from build123d import *

# Parameters (mm, degrees)
SKETCH1_R                                        = 31
BOSS_EXTRUDE1_DEPTH                              = 17.78
CBORE_FOR_3_8_SOCKET_HEAD_CAP_SCREW1_D           = 9.8044
CBORE_FOR_3_8_SOCKET_HEAD_CAP_SCREW1_DEPTH       = 23.8252
CBORE_FOR_3_8_SOCKET_HEAD_CAP_SCREW1_CBORE_D     = 15.875
CBORE_FOR_3_8_SOCKET_HEAD_CAP_SCREW1_CBORE_DEPTH = 9.525
CBORE_FOR_3_8_SOCKET_HEAD_CAP_SCREW1_TIP         = 2.945538927
CHAMFER1_SIZE                                    = 0.762


with BuildPart() as part:
    # Sketch1 → Boss-Extrude1 (new body)
    with BuildSketch(Plane(origin=(0, 0, 0), x_dir=(0, 0, -1), z_dir=(1, 0, 0))):
        Circle(SKETCH1_R)
    extrude(amount=BOSS_EXTRUDE1_DEPTH)

    # CBORE for 3/8 Socket Head Cap Screw1
    with Locations(Plane(origin=(17.78, 0, 0), x_dir=(0, 0, -1), z_dir=(1, 0, 0))):
        with Locations((-15.24, 0), (15.24, 0)):
            CounterBoreHole(CBORE_FOR_3_8_SOCKET_HEAD_CAP_SCREW1_D / 2, CBORE_FOR_3_8_SOCKET_HEAD_CAP_SCREW1_CBORE_D / 2, CBORE_FOR_3_8_SOCKET_HEAD_CAP_SCREW1_CBORE_DEPTH, depth=CBORE_FOR_3_8_SOCKET_HEAD_CAP_SCREW1_DEPTH)
            with Locations((0, 0, -(CBORE_FOR_3_8_SOCKET_HEAD_CAP_SCREW1_DEPTH + CBORE_FOR_3_8_SOCKET_HEAD_CAP_SCREW1_TIP / 2))):  # 118° drill point
                Cone(0, CBORE_FOR_3_8_SOCKET_HEAD_CAP_SCREW1_D / 2, CBORE_FOR_3_8_SOCKET_HEAD_CAP_SCREW1_TIP, mode=Mode.SUBTRACT)

    # Chamfer1
    chamfer1_edges = [part.edges().sort_by_distance(p)[0] for p in [
        (17.78, 0, 23.1775),
        (0, 0, 31),
        (17.78, 0, 31),
        (17.78, 0, -7.3025),
    ]]
    chamfer(chamfer1_edges, length=CHAMFER1_SIZE)


solid = part.part
The model under review builds one solid part; all positions refer to its coordinate system, in mm. A direction names the side the tool comes from. Round coordinates to 2 decimals unless told otherwise and drop trailing zeros. Write each loop counter-clockwise with the first axis right and the second up, starting at its lowest first coordinate (ties: lowest second). Pieces come first, ordered by that corner, then holes. Notation, with made-up numbers: M -16,-4 L 11,-4 A24 cw 11,21 Z; hole C -25,25.25 d7. An arc over 180 degrees is marked long. Answer as CSV lines item,"result". Start each with the question number.
Q1. The part is to be moulded in two halves that separate along Z. For faces 1 (the face through (4.07, 0.216, -20.137)), 2 (the face through (17.78, 0, 0)), 3 (the face through (8.255, 4, 12)), 4 (the face through (8.776, 30.736, 4.036)), say which applies: +Z half, -Z half, draft (parallel to the pull), parting line (faces both ways), or undercut.
Q2. Tool access review of faces 5 (the face through (0, 0, 0)), 6 (the face through (12.698, -3.04, 7.908)): name each direction out of +Z, -Z, +X, -X, +Y, -Y from which nothing blocks a thin tool from reaching the whole face with its end or side.
Q3. Consider section A-A, the plane y = 0. Give the boundary of the cut face in (x, z) (1 decimal).
Q4. Consider section B-B, the plane x = 13.75. Give the boundary of the cut face in (y, z) (1 decimal).
Q5. Wall thickness on line 1 along Y through (x, z) = (14, 0); line 2 along Y through (x, z) = (5.5, -18); line 3 along Z through (x, y) = (7.75, -1): over which ranges is each line inside the solid? List them lowest first.
Q6. Clearance check with flat-ended pins moving along their axes: P1, Ø5, axis at x = 6.5, z = -3.5, coming from the +Y side; P2, Ø2, axis at x = 12, z = 21.5, coming from the +Y side; P3, Ø10, axis at x = 12.5, z = 15, coming from the +Y side. State where each tip first meets the part, or that it passes through.
Q7. Consider section C-C, the plane x = 4. Give the boundary of the cut face in (y, z), then the cut area to 3 significant figures.
Result set:
1,face 1,"undercut"
1,face 2,"draft"
1,face 3,"undercut"
1,face 4,"parting line"
2,face 5,"+Z, -Z, -X, +Y, -Y"
2,face 6,"+X"
3,outline,"M 0,-30.2 L 0.8,-31 L 17,-31 L 17.8,-30.2 L 17.8,-23.9 L 17,-23.2 L 8.3,-23.2 L 8.3,-20.1 L 0,-20.1 Z; M 0,-10.3 L 8.3,-10.3 L 8.3,-7.3 L 17,-7.3 L 17.8,-6.5 L 17.8,6.5 L 17,7.3 L 8.3,7.3 L 8.3,10.3 L 0,10.3 Z; M 0,20.1 L 8.3,20.1 L 8.3,23.2 L 17,23.2 L 17.8,23.9 L 17.8,30.2 L 17,31 L 0.8,31 L 0,30.2 Z"
4,outline,"C 0,0 d62; hole C 0,-15.2 d15.9; hole C 0,15.2 d15.9"
5,line 1,"y = -31 to 31"
5,line 2,"y = -25.24 to -4.05, 4.05 to 25.24"
5,line 3,"z = -30.98 to -20.04, -10.44 to 10.44, 20.04 to 30.98"
6,P1,"stops at y = 30.98"
6,P2,"stops at y = 23.25"
6,P3,"stops at y = 29.34"
7,outline,"C 0,0 d62; hole C 0,-15.24 d9.8; hole C 0,15.24 d9.8"
7,area,"2,870 mm²"
